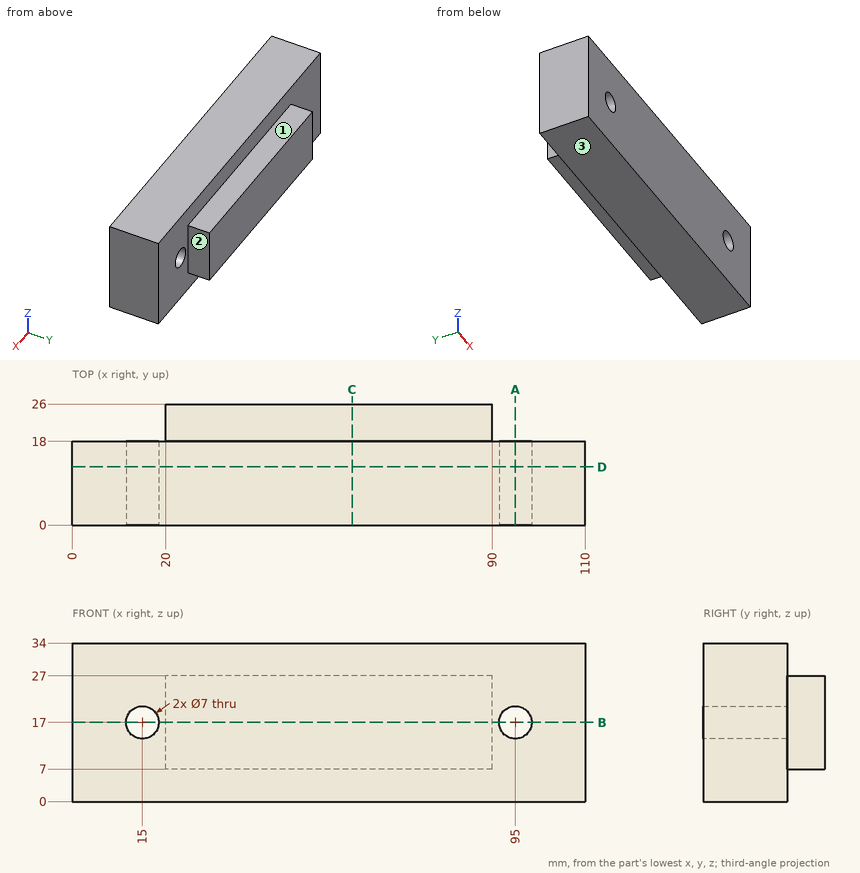
Job drawing, mm, ordinate dimensions from the low corner. One solid piece. A direction names the side the tool comes from. Give positions to 0.01 mm unless a question says otherwise; leave off trailing zeros. Loops run counter-clockwise (first coordinate to the right, second up) from the corner with the lowest first, then second, coordinate; pieces in that order, holes last.
Item 1: Flat gauge pins, fed straight in: pin 1 (6 mm diameter, centred on x = 70, y = 20, fed in from +Z); pin 2 (9 mm diameter, centred on x = 48, y = 24, fed in from -Z); pin 3 (8 mm diameter, centred on x = 95, z = 17, fed in from +Y); pin 4 (6.5 mm diameter, centred on x = 46, y = 24, fed in from +Z). Where does each tip first touch, or does it go through?
Answers follow:
pin 1: stops at z = 34
pin 2: stops at z = 7
pin 3: stops at y = 18
pin 4: stops at z = 27
Item 2: Slice it at D-D, the plane y = 12.5. List the corners of the cut face in (x, z), and give its area (3 significant figures).
Answers follow:
outline: (0, 0) - (110, 0) - (110, 34) - (0, 34) - close; hole circle Ø7 at (15, 17); hole circle Ø7 at (95, 17)
area: 3,660 mm2
Item 3: Slice it at C-C, the plane x = 60. List the corners of the cut face in (y, z).
Answers follow:
outline: (0, 0) - (18, 0) - (18, 7) - (26, 7) - (26, 27) - (18, 27) - (18, 34) - (0, 34) - close
Item 4: Which spindle directions (+Z, -Z, +X, -X, +Y, -Y) get a long thin tool onto all of the face, cutting with end or side? Do the marked faces 1, 2 and 3. Say none if no direction does.
Answers follow:
face 1: +Z, +X, -X, +Y
face 2: +Z, -Z, +X, +Y
face 3: -Z, +X, -X, +Y, -Y
Item 5: Slice it at B-B, the plane z = 17. List the corners of the cut face in (x, y).
Answers follow:
outline: (0, 0) - (11.5, 0) - (11.5, 18) - (0, 18) - close; (18.5, 0) - (91.5, 0) - (91.5, 18) - (90, 18) - (90, 26) - (20, 26) - (20, 18) - (18.5, 18) - close; (98.5, 0) - (110, 0) - (110, 18) - (98.5, 18) - close
Item 6: Drill centre lines: line 1 (X direction, y = 4.75, z = 17); line 2 (X direction, y = 22, z = 14.5); line 3 (Y direction, x = 66, z = 30.5). Where is each one in solid material? Low to high.
Answers follow:
line 1: x = 0 to 11.5, 18.5 to 91.5, 98.5 to 110
line 2: x = 20 to 90
line 3: y = 0 to 18
Item 7: Slice it at A-A, the plane x = 95. List the corners of the cut face in (y, z).
Answers follow:
outline: (0, 0) - (18, 0) - (18, 13.5) - (0, 13.5) - close; (0, 20.5) - (18, 20.5) - (18, 34) - (0, 34) - close
